Part model, mm, in its own coordinate system. Face numbers are marked on the shaded views. A direction names the side the tool comes from. Coordinates: 2 decimals unless noted, no trailing zeros. Order: outer loops, then holes, each group sorted by start corner. A loop starts at its lowest first (then second) coordinate and runs counter-clockwise, first axis right, second up.
1) Tool access for the marked faces 1, 2, 3, 4 and 5: list every direction of +Z, -Z, +X, -X, +Y, -Y with a clear straight run to the whole face (end or side of a thin tool).
2) Cut at D-D (x = 23.5). List the corners of the cut face in (y, z).
3) Pin check, flat tips, straight feed: pin 1 Ø1.5 at (x, y) = (3.5, 6) entering from +Z; pin 2 Ø1 at (y, z) = (-2.5, 18.5) entering from -X; pin 3 Ø9 at (y, z) = (-8.5, 18) entering from -X; pin 4 Ø2.5 at (y, z) = (-8.5, 18) entering from +X. Stop position of each tip, or through.
4) Cut at B-B (y = 4.5). List the corners of the cut face in (x, z), and give its area (3 significant figures).
5) Mould opens along Y. For the marked faces 6, 7, 8 and 9 say: +Y half, -Y half, draft (parallel to the pull), parting line (faces both ways), or undercut.
6) Cut at A-A (z = 21). List the corners of the cut face in (x, y), and give its area (3 significant figures).
7) Cut at C-C (z = 27). List the corners of the cut face in (x, y).
8) Wall check: L1, parallel to X at y = -6.75, z = 46.5; L2, parallel to Z at x = 27, y = 5; L3, parallel to X at y = -10, z = 3.5. Give the ranges that are in metal, low to high.
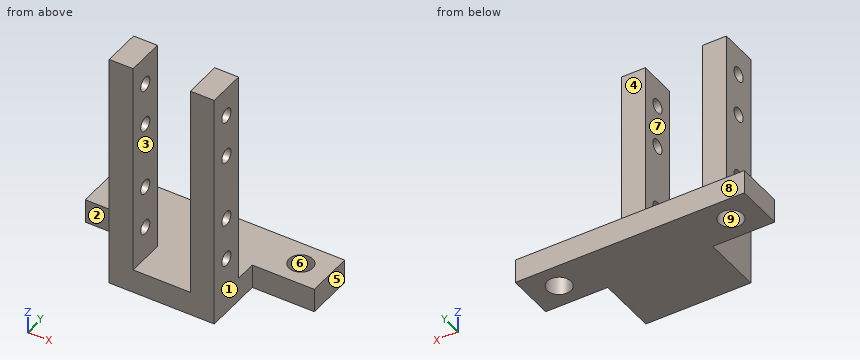
```python
from build123d import *

# Parameters (mm, degrees)
SKETCH_1_R          = 2.5
SKETCH_1_W          = 22
SKETCH_1_H          = 12.5
SKETCH_1_H_2        = 5
EXTRUDE_2_DEPTH     = 5
SKETCH_2_W          = 5
SKETCH_2_H          = 8
EXTRUDE_3_DEPTH     = 45
SKETCH_3_R          = 1.5
CUT_EXTRUDE_1_DEPTH = 45
SKETCH_5_R          = 1.5
CUT_EXTRUDE_2_DEPTH = 45


with BuildPart() as part:
    # 草图1 → 凸台-拉伸2 (new body)
    # profile 1 of 3: a face of its own
    with BuildSketch(Plane.XY):
        Polygon((29.983914209, 11.388739946), (-18.016085791, 11.388739946), (-18.016085791, 1.388739946), (-5.016085791, 1.388739946), (-5.016085791, 6.388739946), (16.983914209, 6.388739946), (16.983914209, 1.388739946), (29.983914209, 1.388739946), align=None)
        with Locations((-12.016085791, 6.388739946)):
            Circle(SKETCH_1_R, mode=Mode.SUBTRACT)
        with Locations((23.983914209, 6.388739946)):
            Circle(SKETCH_1_R, mode=Mode.SUBTRACT)
    # profile 2 of 3: a face of its own
    with BuildSketch(Plane.XY):
        with Locations((5.983914209, -4.861260054)):
            Rectangle(SKETCH_1_W, SKETCH_1_H)
    # profile 3 of 3: a face of its own
    with BuildSketch(Plane.XY):
        with Locations((5.983914209, 3.888739946)):
            Rectangle(SKETCH_1_W, SKETCH_1_H_2)
    extrude(amount=EXTRUDE_2_DEPTH)

    # 草图2 → 凸台-拉伸3 (add)
    with BuildSketch(Plane.XY.offset(5)):
        with Locations((-2.516085791, -7.111260054)):
            Rectangle(SKETCH_2_W, SKETCH_2_H)
        with Locations((14.483914209, -7.111260054)):
            Rectangle(SKETCH_2_W, SKETCH_2_H)
    extrude(amount=EXTRUDE_3_DEPTH)

    # 草图3 → 切除-拉伸1 (cut)
    with BuildSketch(Plane.ZY.offset(5.016085791)):
        with Locations(Location((21, -7.111260054, 0), (0, 0, 270))):
            Circle(SKETCH_3_R)
        with Locations(Location((35, -7.111260054, 0), (0, 0, 270))):
            Circle(SKETCH_3_R)
    extrude(amount=-CUT_EXTRUDE_1_DEPTH, mode=Mode.SUBTRACT)

    # 草图5 → 切除-拉伸2 (cut)
    with BuildSketch(Plane.ZY.offset(5.016085791)):
        with Locations(Location((44, -7.111260054, 0), (0, 0, 270))):
            Circle(SKETCH_5_R)
        with Locations(Location((12, -7.111260054, 0), (0, 0, 270))):
            Circle(SKETCH_5_R)
    extrude(amount=-CUT_EXTRUDE_2_DEPTH, mode=Mode.SUBTRACT)


solid = part.part
```
Geometry check:
1. face 1: +Z, -Z, +X, -Y
1. face 2: +Z, -Z, -X, -Y
1. face 3: +Z, +Y, -Y
1. face 4: +Z, +X, -X, +Y
1. face 5: +Z, -Z, +X, +Y, -Y
2. outline: (1.39, 0) - (3.94, 0) - (3.94, 5) - (1.39, 5) - close; (8.84, 0) - (11.39, 0) - (11.39, 5) - (8.84, 5) - close
3. pin 1: stops at z = 5
3. pin 2: passes through
3. pin 3: stops at x = -5.02
3. pin 4: stops at x = 16.98
4. outline: (-18.02, 0) - (-13.65, 0) - (-13.65, 5) - (-18.02, 5) - close; (-10.38, 0) - (22.35, 0) - (22.35, 5) - (-10.38, 5) - close; (25.62, 0) - (29.98, 0) - (29.98, 5) - (25.62, 5) - close
4. area: 207 mm2
5. face 6: undercut
5. face 7: draft
5. face 8: +Y half
5. face 9: undercut
6. outline: (-5.02, -11.11) - (-0.02, -11.11) - (-0.02, -8.61) - (-5.02, -8.61) - close; (-5.02, -5.61) - (-0.02, -5.61) - (-0.02, -3.11) - (-5.02, -3.11) - close; (11.98, -11.11) - (16.98, -11.11) - (16.98, -8.61) - (11.98, -8.61) - close; (11.98, -5.61) - (16.98, -5.61) - (16.98, -3.11) - (11.98, -3.11) - close
6. area: 50.0 mm2
7. outline: (-5.02, -11.11) - (-0.02, -11.11) - (-0.02, -3.11) - (-5.02, -3.11) - close; (11.98, -11.11) - (16.98, -11.11) - (16.98, -3.11) - (11.98, -3.11) - close
8. L1: x = -5.02 to -0.02, 11.98 to 16.98
8. L2: z = 0 to 5
8. L3: x = -5.02 to 16.98
